from build123d import *

# Parameters (mm, degrees)
SKETCH_1_W          = 28
SKETCH_1_H          = 16
SKETCH_1_R          = 1.5
EXTRUDE_1_DEPTH     = 10
FILLET_1_R          = 3
SKETCH_2_R          = 1.5
EXTRUDE_2_DEPTH     = 0.4
CUT_EXTRUDE_1_DEPTH = 0.1
CUT_EXTRUDE_2_DEPTH = 3
CUT_EXTRUDE_3_DEPTH = 0.1
CUT_EXTRUDE_4_DEPTH = 0.1
SKETCH_7_W          = 2.9
SKETCH_7_H          = 0.1
CUT_EXTRUDE_5_DEPTH = 0.1
SKETCH_8_W          = 2.9
SKETCH_8_H          = 0.1
CUT_EXTRUDE_6_DEPTH = 0.1
EXTRUDE_3_DEPTH     = 4.5
SKETCH_11_W         = 10
SKETCH_11_H         = 0.8
EXTRUDE_4_DEPTH     = 6.5
SKETCH_12_R         = 0.75
CUT_EXTRUDE_7_DEPTH = 53.388166603
FILLET_2_R          = 1
SKETCH_13_R         = 0.75
CUT_EXTRUDE_8_DEPTH = 2
EXTRUDE_6_DEPTH     = 4.5
EXTRUDE_7_DEPTH     = 4.5
CUT_EXTRUDE_9_DEPTH = 0.13


with BuildPart() as part:
    # 草图1 → 凸台-拉伸1 (new body)
    with BuildSketch(Plane(origin=(0, 0, 0), x_dir=(0, 0, -1), z_dir=(1, 0, 0))):
        Rectangle(SKETCH_1_W, SKETCH_1_H)
        with Locations((11, -5)):
            Circle(SKETCH_1_R, mode=Mode.SUBTRACT)
        with Locations((-11, 5)):
            Circle(SKETCH_1_R, mode=Mode.SUBTRACT)
    extrude(amount=EXTRUDE_1_DEPTH)

    # 圆角1
    fillet_1_edges = [part.edges().sort_by_distance(p)[0] for p in [
        (5, 8, 14),
        (5, 8, -14),
        (5, -8, -14),
        (5, -8, 14),
    ]]
    fillet(fillet_1_edges, radius=FILLET_1_R)

    # 草图2 → 凸台-拉伸2 (add)
    # profile 1 of 2: a face of its own
    with BuildSketch(Plane(origin=(10, 0, 0), x_dir=(0, 0, -1), z_dir=(1, 0, 0))):
        with BuildLine():
            Line((13.5, -5), (13.5, -2.1))
            Line((13.5, -2.1), (11, -2.1))
            ThreePointArc((11, -2.1), (8.949390335, -2.949390335), (8.1, -5))
            Line((8.1, -5), (8.1, -7.5))
            Line((8.1, -7.5), (11, -7.5))
            ThreePointArc((11, -7.5), (12.767766953, -6.767766953), (13.5, -5))
        make_face()
        with Locations((11, -5)):
            Circle(SKETCH_2_R, mode=Mode.SUBTRACT)
    # profile 2 of 2: a face of its own
    with BuildSketch(Plane(origin=(10, 0, 0), x_dir=(0, 0, -1), z_dir=(1, 0, 0))):
        with BuildLine():
            Line((-11, 2.1), (-13.5, 2.1))
            Line((-13.5, 2.1), (-13.5, 5))
            ThreePointArc((-13.5, 5), (-12.767766953, 6.767766953), (-11, 7.5))
            Line((-11, 7.5), (-8.1, 7.5))
            Line((-8.1, 7.5), (-8.1, 5))
            ThreePointArc((-8.1, 5), (-8.949390335, 2.949390335), (-11, 2.1))
        make_face()
        with Locations((-11, 5)):
            Circle(SKETCH_2_R, mode=Mode.SUBTRACT)
    extrude(amount=EXTRUDE_2_DEPTH)

    # 草图3 → 切除-拉伸1 (cut)
    with BuildSketch(Plane.ZY):
        with BuildLine():
            Line((-13.5, -2.1), (-11, -2.1))
            ThreePointArc((-11, -2.1), (-8.949390335, -2.949390335), (-8.1, -5))
            Line((-8.1, -5), (-8.1, -7.5))
            Line((-8.1, -7.5), (-8.1, -8))
            Line((-8.1, -8), (-8.2, -8))
            Line((-8.2, -8), (-8.2, -7.5))
            Line((-8.2, -7.5), (-8.2, -5))
            ThreePointArc((-8.2, -5), (-9.020101013, -3.020101013), (-11, -2.2))
            Line((-11, -2.2), (-13.5, -2.2))
            Line((-13.5, -2.2), (-14, -2.2))
            Line((-14, -2.2), (-14, -2.1))
            Line((-14, -2.1), (-13.5, -2.1))
        make_face()
        with BuildLine():
            Line((13.5, 2.1), (11, 2.1))
            ThreePointArc((11, 2.1), (8.949390335, 2.949390335), (8.1, 5))
            Line((8.1, 5), (8.1, 7.5))
            Line((8.1, 7.5), (8.1, 8))
            Line((8.1, 8), (8.2, 8))
            Line((8.2, 8), (8.2, 7.5))
            Line((8.2, 7.5), (8.2, 5))
            ThreePointArc((8.2, 5), (9.020101013, 3.020101013), (11, 2.2))
            Line((11, 2.2), (13.5, 2.2))
            Line((13.5, 2.2), (14, 2.2))
            Line((14, 2.2), (14, 2.1))
            Line((14, 2.1), (13.5, 2.1))
        make_face()
    extrude(amount=-CUT_EXTRUDE_1_DEPTH, mode=Mode.SUBTRACT)

    # 草图4 → 切除-拉伸2 (cut)
    with BuildSketch(Plane(origin=(0, 8, 0), x_dir=(1, 0, 0), z_dir=(0, 1, 0))):
        Polygon((0, -8.2), (3.1, -8.2), (3.1, 14), (3, 14), (3, -8.1), (0, -8.1), align=None)
    extrude(amount=-CUT_EXTRUDE_2_DEPTH, mode=Mode.SUBTRACT)

    # 草图5 → 切除-拉伸3 (cut)
    with BuildSketch(Plane(origin=(0, 0, -14), x_dir=(-1, 0, 0), z_dir=(0, 0, -1))):
        Polygon((-3, 5), (-3, -2.1), (-0.1, -2.1), (-0.1, -2.2), (-3.1, -2.2), (-3.1, 5), align=None)
    extrude(amount=-CUT_EXTRUDE_3_DEPTH, mode=Mode.SUBTRACT)

    # 草图6 → 切除-拉伸4 (cut)
    with BuildSketch(Plane.ZY.offset(-3.1)):
        with BuildLine():
            Line((-8.2, -8), (11, -8))
            ThreePointArc((11, -8), (13.121320344, -7.121320344), (14, -5))
            Line((14, -5), (14, 2.1))
            Line((14, 2.1), (14, 2.2))
            Line((14, 2.2), (13.9, 2.2))
            Line((13.9, 2.2), (13.9, 2.1))
            Line((13.9, 2.1), (13.9, -5))
            ThreePointArc((13.9, -5), (13.050609665, -7.050609665), (11, -7.9))
            Line((11, -7.9), (-8.2, -7.9))
            Line((-8.2, -7.9), (-8.2, -8))
        make_face()
    extrude(amount=CUT_EXTRUDE_4_DEPTH, mode=Mode.SUBTRACT)

    # 草图7 → 切除-拉伸5 (cut)
    with BuildSketch(Plane.XY.offset(14)):
        with Locations((1.55, 2.15)):
            Rectangle(SKETCH_7_W, SKETCH_7_H)
    extrude(amount=-CUT_EXTRUDE_5_DEPTH, mode=Mode.SUBTRACT)

    # 草图8 → 切除-拉伸6 (cut)
    with BuildSketch(Plane.XZ.offset(8)):
        with Locations((1.55, -8.15)):
            Rectangle(SKETCH_8_W, SKETCH_8_H)
    extrude(amount=-CUT_EXTRUDE_6_DEPTH, mode=Mode.SUBTRACT)

    # 草图10 → 凸台-拉伸3 (add)
    with BuildSketch(Plane.ZY.offset(-3.1)):
        Polygon((-2.6, -8), (-2.6, -10), (49.4, -10), (49.4, -9.5), (-2.1, -9.5), (-2.1, -8), align=None)
        with BuildLine():
            Line((11, -8.08), (11, -8))
            Line((11, -8), (8.2, -8))
            Line((8.2, -8), (8.2, -8.08))
            ThreePointArc((8.2, -8.08), (9.6, -9.48), (11, -8.08))
        make_face()
    extrude(amount=-EXTRUDE_3_DEPTH)

    # 草图11 → 凸台-拉伸4 (add)
    with BuildSketch(Plane.ZY.offset(-2)):
        with Locations((-19, 3.6)):
            Rectangle(SKETCH_11_W, SKETCH_11_H)
        with Locations((-19, -2.2)):
            Rectangle(SKETCH_11_W, SKETCH_11_H)
        Polygon((-1, 8), (-1, 10.5), (-10.5, 10.5), (-10.5, 9.7), (-1.8, 9.7), (-1.8, 8), align=None)
    extrude(amount=-EXTRUDE_4_DEPTH)

    # 草图12 → 切除-拉伸7 (cut, through all)
    with BuildSketch(Plane(origin=(0, 4, 0), x_dir=(1, 0, 0), z_dir=(0, 1, 0))):
        with Locations(Location((5.25, 20, 0), (0, 0, 270))):
            Circle(SKETCH_12_R)
        Polygon((2, 17.5), (3, 17.5), (3, 22), (4.154700538, 24), (3, 24), (2, 24), align=None)
        Polygon((8.5, 24), (8.5, 17.5), (7.5, 17.5), (7.5, 22), (6.345299462, 24), (7.5, 24), align=None)
    extrude(amount=-CUT_EXTRUDE_7_DEPTH, mode=Mode.SUBTRACT)

    # 圆角2
    fillet_2_edges = [part.edges().sort_by_distance(p)[0] for p in [
        (5.35, -10, -2.6),
        (5.35, -9.5, -2.1),
        (5.25, 9.7, -1.8),
        (5.25, 10.5, -1),
    ]]
    fillet(fillet_2_edges, radius=FILLET_2_R)

    # 草图13 → 切除-拉伸8 (cut)
    with BuildSketch(Plane(origin=(0, 10.5, 0), x_dir=(1, 0, 0), z_dir=(0, 1, 0))):
        with Locations(Location((5.25, 6.5, 0), (0, 0, 270))):
            Circle(SKETCH_13_R)
        Polygon((8.5, 10.5), (6.345299462, 10.5), (7.5, 8.5), (7.5, 4), (8.5, 4), align=None)
        Polygon((3, 4), (2, 4), (2, 10.5), (4.154700538, 10.5), (3, 8.5), align=None)
    extrude(amount=-CUT_EXTRUDE_8_DEPTH, mode=Mode.SUBTRACT)

    # 草图10<5> → 凸台-拉伸6 (add)
    with BuildSketch(Plane.ZY.offset(-3.1)):
        with BuildLine():
            Line((8.223055296, -8.333028221), (-2.1, -9.5))
            Line((-2.1, -9.5), (2.351181411, -9.5))
            Line((2.351181411, -9.5), (8.408603451, -8.815237556))
            ThreePointArc((8.408603451, -8.815237556), (8.293391543, -8.582766687), (8.223055296, -8.333028221))
        make_face()
        with BuildLine():
            ThreePointArc((11, -8.08), (10.981240109, -8.308420142), (10.925463198, -8.53071866))
            Line((10.925463198, -8.53071866), (49.130220738, -4.211854469))
            Line((49.130220738, -4.211854469), (49.074055873, -3.715018975))
            Line((49.074055873, -3.715018975), (11.77713938, -7.9312561))
            Line((11.77713938, -7.9312561), (11.77713938, -7.9812561))
            Line((11.77713938, -7.9812561), (11, -8.069107971))
            Line((11, -8.069107971), (11, -8.08))
        make_face()
    extrude(amount=-EXTRUDE_6_DEPTH)

    # 草图10<6> → 凸台-拉伸7 (add)
    with BuildSketch(Plane.ZY.offset(-3.1)):
        Polygon((3.75, -10), (-2.6, -10), (49.2111008, -14.428299214), (49.257152, -13.889500171), (9.6, -10.5), align=None)
    extrude(amount=-EXTRUDE_7_DEPTH)

    # 草图14 → 切除-拉伸9 (cut)
    with BuildSketch(Plane.ZY.offset(-3.1)):
        with BuildLine():
            Line((39.135085265, -4.838571826), (49.072235928, -3.715224711))
            ThreePointArc((49.072235928, -3.715224711), (49.444709047, -9.069072224), (49.263942313, -14.432815582))
            Line((49.263942313, -14.432815582), (39.300269083, -13.58121958))
            ThreePointArc((39.300269083, -13.58121958), (39.445530044, -9.205590645), (39.135085265, -4.838571826))
        make_face()
    extrude(amount=-CUT_EXTRUDE_9_DEPTH, mode=Mode.SUBTRACT)


solid = part.part
Source: CAD feature listing. Evaluate the final solid. Frame: model axes, mm. A direction names the side the tool comes from. Coordinates: 2 decimals unless noted, no trailing zeros. Loops run counter-clockwise (first coordinate to the right, second up) from the corner with the lowest first, then second, coordinate; pieces in that order, holes last. Notation, with made-up numbers: (-35, 53) - (-8, 53) arc R22 ccw to (-8, 92) - close; hole circle Ø4 at (48.25, 6). An arc over 180 degrees is marked (long way). Return JSON: item names as keys, results as strings.
Q1. Material intervals for line 1 along X through (y, z) = (10, -6.5); line 2 along Y through (x, z) = (5, 28.5); line 3 along Y through (x, z) = (8, 11), sorted ascending.
Results:
{"line 1": "3 to 4.5, 6 to 7.5", "line 2": "-12.66 to -12.12, -10 to -9.5, -6.54 to -6.04", "line 3": "-8 to 3.5, 6.5 to 8"}
Q2. Section B-B, the plane z = -6.5. Return loops of the section in (x, y).
Results:
{"outline": "(0, -8) - (3, -8) - (3, -7.9) - (3.1, -7.9) - (3.1, -8) - (10, -8) - (10, 8) - (3.1, 8) - (3.1, 5) - (3, 5) - (3, 8) - (0, 8) - close; (3, 9.7) - (4.5, 9.7) - (4.5, 10.5) - (3, 10.5) - close; (6, 9.7) - (7.5, 9.7) - (7.5, 10.5) - (6, 10.5) - close"}
Q3. Mould query, pull axis Z, two halves, no side actions, for faces 5 (the flat face through (1, 8, -1)), 6 (the flat face through (5.318, -8.873, 3.444)), 7 (the cylindrical face through (10.197, 6.748, 12.787)). Classes: released by +Z, released by -Z, zero draft, split by the parting line, or undercut.
Results:
{"face 5": "zero draft", "face 6": "undercut", "face 7": "released by +Z"}
Q4. Section C-C, the plane z = 15.5. Return loops of the section in (x, y), plus the area to 3 significant figures.
Results:
{"outline": "(3.1, -11.55) - (7.6, -11.55) - (7.6, -11) - (3.1, -11) - close; (3.1, -10) - (7.6, -10) - (7.6, -9.5) - (3.1, -9.5) - close; (3.1, -8.01) - (7.6, -8.01) - (7.6, -7.51) - (3.1, -7.51) - close", "area": "6.96 mm2"}
Q5. Section A-A, the plane z = -20. Return loops of the section in (x, y).
Results:
{"outline": "(3, -2.6) - (4.5, -2.6) - (4.5, -1.8) - (3, -1.8) - close; (3, 3.2) - (4.5, 3.2) - (4.5, 4) - (3, 4) - close; (6, -2.6) - (7.5, -2.6) - (7.5, -1.8) - (6, -1.8) - close; (6, 3.2) - (7.5, 3.2) - (7.5, 4) - (6, 4) - close"}
Q6. Access query for faces 1 (the flat face through (5, -1.8, -18)), 2 (the flat face through (5, -2.6, -18)), 3 (the cylindrical face through (10.2, -2.9, -9)), 4 (the flat face through (0, -6.3, -12.3)). Directions: +Z, -Z, +X, -X, +Y, -Y. A direction counts if a zero-diameter tool reaches every point of the face in a straight line with its end or side. Return the directions, or none.
Results:
{"face 1": "-Z, +X, -X", "face 2": "-Z, +X, -X, -Y", "face 3": "+Z, +X, +Y", "face 4": "+Z, -Z, -X, +Y, -Y"}
Q7. Contact query for flat-ended pins moving along their axis: P1, Ø1, axis at x = 7.5, y = -0.5, coming from the +Z side; P2, Ø2, axis at x = 6.5, z = -4.5, coming from the -Y side; P3, Ø1.5, axis at y = -11.5, z = 20, coming from the +X side. Output: stop coordinate, or through.
Results:
{"P1": "z = 14", "P2": "y = -8", "P3": "x = 7.6"}
